Can you work these out from the drawing? Everything is in mm from the part's minimum corner. A direction names the side the tool comes from. Coordinates: 2 decimals unless noted, no trailing zeros. Write each loop counter-clockwise with the first axis right and the second up, starting at its lowest first coordinate (ties: lowest second). Pieces come first, ordered by that corner, then holes. Notation, with made-up numbers: M 80,23.5 L 97,23.5 A12 cw 97,46.5 Z; hole C 5,0 d10. An arc over 180 degrees is marked long. Write each question's results on one line, items separated by ' | '. Start each with the question number.
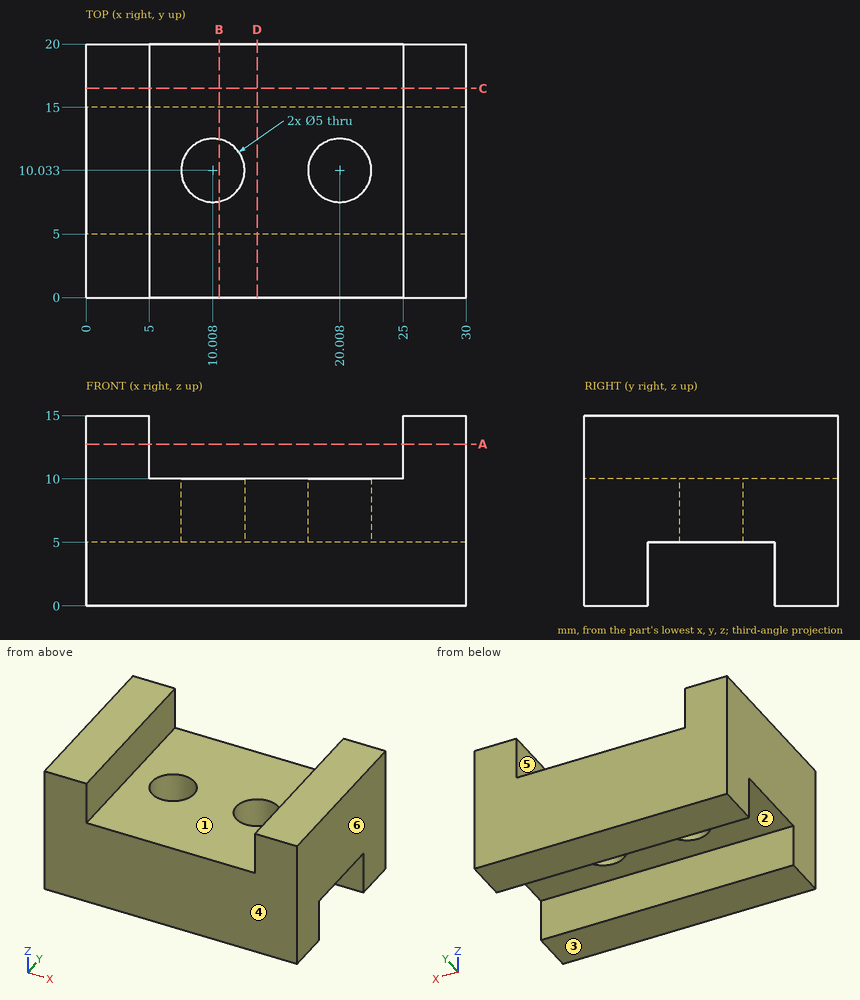
1) I want a section at B-B, the plane x = 10.5. Write out the boundary of the cut face in (y, z).
2) I want a section at C-C, the plane y = 16.5. Write out the boundary of the cut face in (x, z), then the cut area to 3 significant figures.
3) We'd pull the mould along X, two halves only. Please class the marked faces 4, 5 and 6: pulls with the +X half, pulls with the -X half, needs draft (parallel to the pull), parting line crosses it, or undercut.
4) For the marked faces 1, 2 and 3, which set-ups out of +Z, -Z, +X, -X, +Y, -Y let a thin tool reach every point of the face, with its end or its side?
5) Please list where these lines run through material, in increasing order: line 1 (Y direction, x = 7, z = 3.5); line 2 (X direction, y = 13.25, z = 14.5); line 3 (Z direction, x = 23, y = 14.25). Write a range as [from, to].
6) I want a section at D-D, the plane x = 13.5. Write out the boundary of the cut face in (y, z).
7) For pin 1 Ø3 at (x, y) = (10.01, 10.03) entering from -Z; pin 2 Ø10 at (x, y) = (13, 8.5) entering from +Z, each with a flat end and sliding along its axis, tell me the tip position at first contact or that it passes through.
8) I want a section at A-A, the plane z = 12.75. Write out the boundary of the cut face in (x, y).
Output:
1) outline: M 0,0 L 5,0 L 5,5 L 7.58,5 L 7.58,10 L 0,10 Z; M 12.48,5 L 15,5 L 15,0 L 20,0 L 20,10 L 12.48,10 Z
2) outline: M 0,0 L 30,0 L 30,15 L 25,15 L 25,10 L 5,10 L 5,15 L 0,15 Z | area: 350 mm2
3) face 4: needs draft | face 5: undercut | face 6: pulls with the +X half
4) face 1: +Z, +Y, -Y | face 2: -Z, +X, -X | face 3: -Z, +X, -X, +Y, -Y
5) line 1: y = [0, 5], [15, 20] | line 2: x = [0, 5], [25, 30] | line 3: z = [5, 10]
6) outline: M 0,0 L 5,0 L 5,5 L 15,5 L 15,0 L 20,0 L 20,10 L 0,10 Z
7) pin 1: passes through | pin 2: stops at z = 10
8) outline: M 0,0 L 5,0 L 5,20 L 0,20 Z; M 25,0 L 30,0 L 30,20 L 25,20 Z
